from build123d import *

# Parameters (mm, degrees)
SKETCH1_W                   = 18
SKETCH1_H                   = 14
BOSS_EXTRUDE1_DEPTH         = 2
SKETCH2_R                   = 7
BOSS_EXTRUDE2_DEPTH         = 2
M12X1_25_TAPPED_HOLE1_D     = 10.8
M12X1_25_TAPPED_HOLE1_DEPTH = 8.75
M12X1_25_TAPPED_HOLE1_TIP   = 3.244647343
CHAMFER6_SIZE               = 5
CHAMFER7_SIZE               = 1


with BuildPart() as part:
    # Sketch1 → Boss-Extrude1 (new body)
    with BuildSketch(Plane.XY):
        Rectangle(SKETCH1_W, SKETCH1_H)
    extrude(amount=BOSS_EXTRUDE1_DEPTH)

    # Sketch2 → Boss-Extrude2 (add)
    with BuildSketch(Plane.XY.offset(2)):
        with Locations(Location((0, 0, 0), (0, 0, 270))):
            Circle(SKETCH2_R)
    extrude(amount=BOSS_EXTRUDE2_DEPTH)

    # M12x1.25 Tapped Hole1
    with Locations(Plane.XY.offset(4)):
        with Locations((0, 0)):
            Hole(M12X1_25_TAPPED_HOLE1_D / 2, depth=M12X1_25_TAPPED_HOLE1_DEPTH)
            with Locations((0, 0, -(M12X1_25_TAPPED_HOLE1_DEPTH + M12X1_25_TAPPED_HOLE1_TIP / 2))):  # 118° drill point
                Cone(0, M12X1_25_TAPPED_HOLE1_D / 2, M12X1_25_TAPPED_HOLE1_TIP, mode=Mode.SUBTRACT)

    # Chamfer6
    chamfer6_edges = [part.edges().sort_by_distance(p)[0] for p in [
        (9, -7, 1),
        (-9, -7, 1),
    ]]
    chamfer(chamfer6_edges, length=CHAMFER6_SIZE)

    # Chamfer7
    chamfer7_edges = [part.edges().sort_by_distance(p)[0] for p in [
        (-9, 7, 1),
        (9, 7, 1),
    ]]
    chamfer(chamfer7_edges, length=CHAMFER7_SIZE)


solid = part.part
Part model, mm, in its own coordinate system. A direction names the side the tool comes from. Give positions to 0.01 mm unless a question says otherwise; leave off trailing zeros. Loops run counter-clockwise (first coordinate to the right, second up) from the corner with the lowest first, then second, coordinate; pieces in that order, holes last.
(1) Drill centre lines: line 1 along Y through (x, z) = (0, 0.8); line 2 along X through (y, z) = (4.5, 2.85); line 3 along X through (y, z) = (1.5, 2.55). Where is each one in solid material? Low to high.
Return value:
line 1: y = -7 to -5.4, 5.4 to 7
line 2: x = -5.36 to -2.98, 2.98 to 5.36
line 3: x = -6.84 to -5.19, 5.19 to 6.84
(2) Band-saw the part on B-B (x = 1.75). Write the cut outline in (y, z).
Return value:
outline: (-7, 0) - (-5.11, 0) - (-5.11, 4) - (-6.78, 4) - (-6.78, 2) - (-7, 2) - close; (5.11, 0) - (7, 0) - (7, 2) - (6.78, 2) - (6.78, 4) - (5.11, 4) - close
(3) Band-saw the part on D-D (z = 3.2). Write the cut outline in (x, y).
Return value:
outline: circle Ø14 at (0, 0); hole circle Ø10.8 at (0, 0)
(4) Pull direction Y, two halves, no side cores. Call faces 1 (the flat face through (6, -5, 1)), 2 (the flat face through (-7, 3, 2)), 3 (the flat face through (8.5, 6.5, 1)), 4 (the cylindrical face through (1.17, -5.27, 1.97)): pulls with the +Y half, pulls with the -Y half, needs draft (parallel to the pull), parting line crosses it, or undercut.
Return value:
face 1: pulls with the -Y half
face 2: needs draft
face 3: pulls with the +Y half
face 4: undercut
(5) Band-saw the part on C-C (z = 1.1). Write the cut outline in (x, y).
Return value:
outline: (-9, -2) - (-4, -7) - (4, -7) - (9, -2) - (9, 6) - (8, 7) - (-8, 7) - (-9, 6) - close; hole circle Ø10.8 at (0, 0)
(6) Pin check, flat tip, straight feed: pin 1 (1.5 mm diameter, centred on y = -1, z = 3, fed in from +X). Stop position of the tip, or through.
Return value:
pin 1: stops at x = 7
(7) 3-axis set-ups, long thin cutter, end or side, ignore diameter. For faces 5 (the flat face through (-4, -4, 4)), 6 (the cylindrical face through (-6.834, 1.517, 2.986)), 7 (the flat face through (7, 2, 2)): which of +Z, -Z, +X, -X, +Y, -Y reach the whole face in a straight line?
Return value:
face 5: +Z, +X, -X, +Y, -Y
face 6: +Z
face 7: +Z, +X
(8) Band-saw the part on A-A (y = 0). Write the cut outline in (x, z), and give its area (3 significant figures).
Return value:
outline: (-9, 0) - (-5.4, 0) - (-5.4, 4) - (-7, 4) - (-7, 2) - (-9, 2) - close; (5.4, 0) - (9, 0) - (9, 2) - (7, 2) - (7, 4) - (5.4, 4) - close
area: 20.8 mm2
